from build123d import *

# Parameters (mm, degrees)
F0_W     = 65
F0_H     = 12.5
F1_DEPTH = 50
F3_DEPTH = 45.5
F4_W     = 5.1
F4_H     = 5.1
F5_DEPTH = 1.2
F6_R     = 1
F7_W     = 15
F7_H     = 1.1837528777
F8_DEPTH = 2
F9_R     = 1


# Not quite as in the source:
# - a pattern or mirror of a feature is missing from the dataset's text; its kind, count and spacing are read off the source's solid


with BuildPart() as f1:
    # F0 (on Right) → F1 (new body, symmetric)
    with BuildSketch(Plane.YZ):
        Rectangle(F0_W, F0_H)
    extrude(amount=F1_DEPTH, both=True)

    # F2 (on Right) → F3 (cut, symmetric)
    with BuildSketch(Plane.YZ):
        Polygon((-32.5, 6.25), (-32.5, 0), (-25.5, 0), (-25.5, -3.1976206858), (15.3335404618, -3.1976206858), (20.620416518, -6.25), (32.5, -6.25), (32.5, 6.25), align=None)
    extrude(amount=F3_DEPTH, both=True, mode=Mode.SUBTRACT)

    # F4 (on face) → F5 (cut)
    with BuildSketch(Plane.XY):
        with Locations((-39.95, -29.0152)):
            Rectangle(F4_W, F4_H)
    f5 = extrude(amount=-F5_DEPTH, mode=Mode.SUBTRACT)

    # F5_copies: F5 across plane
    add(f5.mirror(Plane(origin=(0, 0, 0), x_dir=(0, 0, 1), z_dir=(1, 0, 0))), mode=Mode.SUBTRACT)

    # F6
    f6_edges = [f1.edges().sort_by_distance(p)[0] for p in [
        (-47.75, -32.5, 6.25),
        (47.75, -32.5, 6.25),
        (-50, 0, 6.25),
        (-47.75, 32.5, 6.25),
        (47.75, 32.5, 6.25),
        (50, 0, 6.25),
        (-50, -32.5, 0),
        (50, -32.5, 0),
        (0, -32.5, -6.25),
        (50, 0, -6.25),
        (50, 32.5, 0),
        (-50, 0, -6.25),
        (-50, 32.5, 0),
        (-47.75, 32.5, -6.25),
        (47.75, 32.5, -6.25),
    ]]
    fillet(f6_edges, radius=F6_R)

    # F7 (on face) → F8 (cut)
    with BuildSketch(Plane.XZ.offset(32.5)):
        with Locations((0, -0.5918764388)):
            Rectangle(F7_W, F7_H)
    extrude(amount=-F8_DEPTH, mode=Mode.SUBTRACT)

    # F9
    f9_edges = [f1.edges().sort_by_distance(p)[0] for p in [
        (0, -30.5, -1.183753),
    ]]
    fillet(f9_edges, radius=F9_R)


solid = f1.part
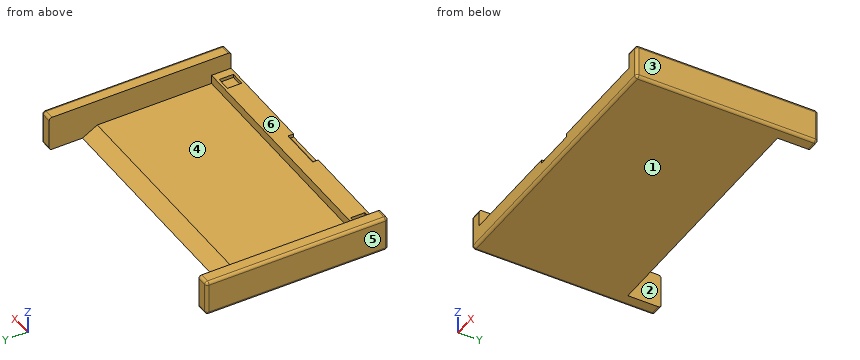
The model under review builds one solid part; all positions refer to its coordinate system, in mm. Face numbers are marked on the shaded views. A direction names the side the tool comes from. Give positions to 0.01 mm unless a question says otherwise; leave off trailing zeros. Write each loop counter-clockwise with the first axis right and the second up, starting at its lowest first coordinate (ties: lowest second). Pieces come first, ordered by that corner, then holes.
1. Add section C-C, the plane x = 3.5. Write out the cut boundary in (y, z), plus the area to 3 significant figures.
2. Draft analysis for pull direction X (two halves, no side actions). For the marked faces 1, 2 and 3, state which applies: +X half, -X half, draft (parallel to the pull), parting line (faces both ways), or undercut.
3. Add section D-D, the plane z = -4.25. Write out the cut boundary in (x, y).
4. Wall thickness on L1, parallel to X at y = -1, z = 3.75; L2, parallel to Z at x = -22.5, y = -18.5; L3, parallel to Y at x = 4, z = -1.5: over which ranges is each line inside the solid? List them lowest first.
5. For P1, Ø0.6, axis at y = -32, z = -0.5, coming from the -X side; P2, Ø5.5, axis at x = 39.5, y = -28, coming from the +Z side; P3, Ø1.6, axis at x = -14.5, z = -2, coming from the +Y side, all flat-tipped, find the tip position at first contact; note any pin that passes through.
6. Tool access review of the marked faces 4, 5 and 6: name each direction out of +Z, -Z, +X, -X, +Y, -Y from which nothing blocks a thin tool from reaching the whole face with its end or side.
7. Add section A-A, the plane z = 4.25. Write out the cut boundary in (x, y).
8. Add section B-B, the plane y = -9. Write out the cut boundary in (x, z).
Worked answers:
1. outline: (-32.5, -5.25) arc R1 ccw to (-31.5, -6.25) - (20.62, -6.25) - (15.33, -3.2) - (-25.5, -3.2) - (-25.5, 0) - (-30.5, 0) - (-30.5, -0.18) arc R1 cw to (-31.5, -1.18) - (-32.5, -1.18) - close
1. area: 174 mm2
2. face 1: draft
2. face 2: undercut
2. face 3: +X half
3. outline: (-50, -31.5) arc R1 ccw to (-49, -32.5) - (49, -32.5) arc R1 ccw to (50, -31.5) - (50, 31.5) arc R1 ccw to (49, 32.5) - (45.5, 32.5) - (45.5, 17.16) - (-45.5, 17.16) - (-45.5, 32.5) - (-49, 32.5) arc R1 ccw to (-50, 31.5) - close
4. L1: x = -50 to -45.5, 45.5 to 50
4. L2: z = -6.25 to -3.2
4. L3: y = -32.5 to -25.5
5. P1: stops at x = -49.98
5. P2: stops at z = 0
5. P3: stops at y = -25.5
6. face 4: +Z, +Y
6. face 5: +Z, -Z, -X, +Y, -Y
6. face 6: +Z, +Y, -Y
7. outline: (-50, -31.5) arc R1 ccw to (-49, -32.5) - (-45.5, -32.5) - (-45.5, 32.5) - (-49, 32.5) arc R1 ccw to (-50, 31.5) - close; (45.5, -32.5) - (49, -32.5) arc R1 ccw to (50, -31.5) - (50, 31.5) arc R1 ccw to (49, 32.5) - (45.5, 32.5) - close
8. outline: (-50, -5.25) arc R1 ccw to (-49, -6.25) - (49, -6.25) arc R1 ccw to (50, -5.25) - (50, 5.25) arc R1 ccw to (49, 6.25) - (45.5, 6.25) - (45.5, -3.2) - (-45.5, -3.2) - (-45.5, 6.25) - (-49, 6.25) arc R1 ccw to (-50, 5.25) - close
